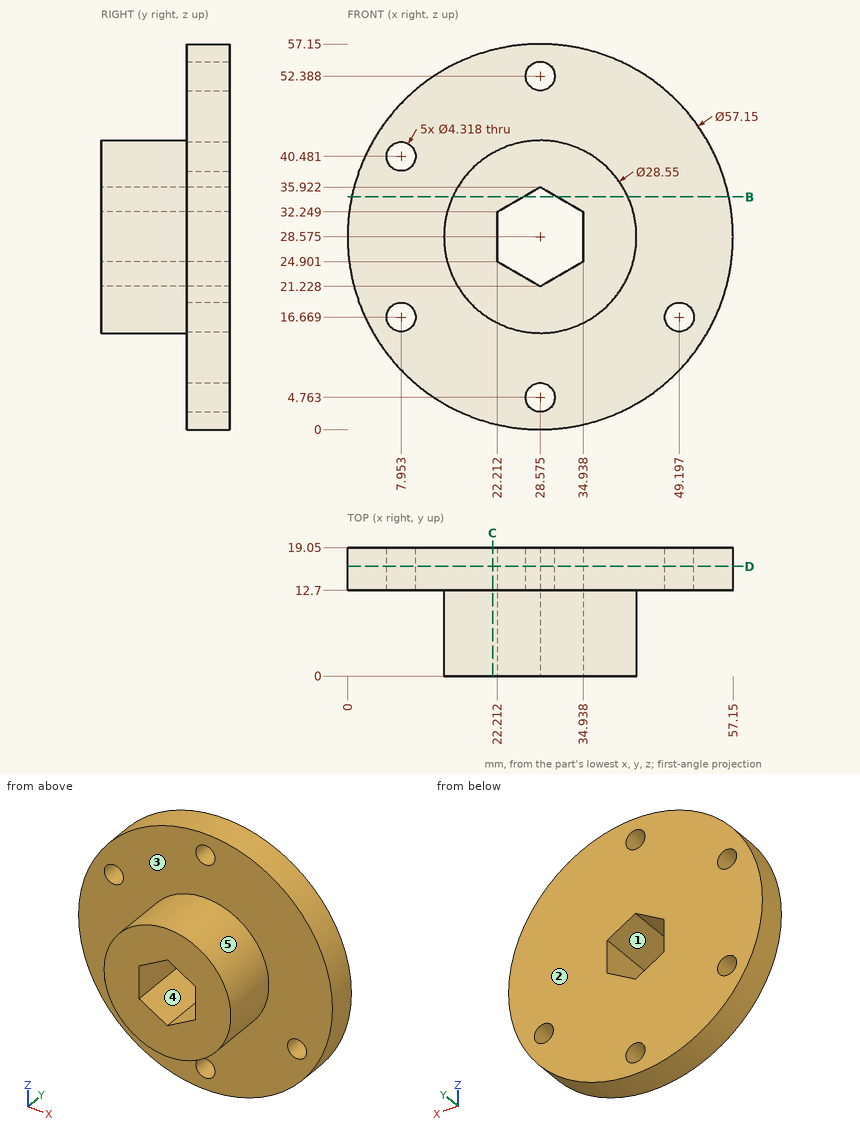
For this review, use the dimensioned drawing (mm, ordinates from the lowest corner) and the shaded views. A direction names the side the tool comes from. Coordinates: 2 decimals unless noted, no trailing zeros. Loops run counter-clockwise (first coordinate to the right, second up) from the corner with the lowest first, then second, coordinate; pieces in that order, holes last. Notation, with made-up numbers: (45, 34) - (53, 34) arc R29 cw to (53, 63) - close; hole circle Ø9 at (-35, -21.75). An arc over 180 degrees is marked (long way). Use one line per item in the form item = value. Start each with the question number.
1) Take a section at B-B (z = 34.5). State the section outline as (x, y) points.
2) Take a section at C-C (x = 21.5). State the section outline as (y, z) points.
3) To check wall thickness, follow probe 1 along X at (y, z) = (1.25, 30); probe 2 along X at (y, z) = (17.5, 29); probe 3 along Y at (x, z) = (30, 44). State the ranges of each line that lie inside material, in increasing order. Write a range as from..to.
4) Take a section at D-D (y = 16.25). State how many separate pieces and enclosed holes the cut face has, plus the area to 3 significant figures.
5) For the marked faces 1 and 2, list the 3-axis set-ups (+Z, -Z, +X, -X, +Y, -Y) from which the entire face can be reached by the end or side of a thin tool; tool diameter is ignored.
6) For pin 1 (1 mm diameter, centred on x = 24, y = 8, fed in from +Z) (1 decimal); pin 2 (1 mm diameter, centred on y = 8, z = 42, fed in from +X) (1 decimal); pin 3 (3 mm diameter, centred on x = 34.5, y = 6.5, fed in from -Z), all flat-tipped, find the tip position at first contact; note any pin that passes through.
7) Draft analysis for pull direction Z (two halves, no side actions). For the marked faces 3, 4 and 5, state which applies: released by +Z, released by -Z, zero draft, split by the parting line, or undercut.
From the geometry:
q1.outline = (0.62, 12.7) - (15.59, 12.7) - (15.59, 0) - (26.11, 0) - (26.11, 19.05) - (0.62, 19.05) - close; (31.04, 0) - (41.56, 0) - (41.56, 12.7) - (56.53, 12.7) - (56.53, 19.05) - (31.04, 19.05) - close
q2.outline = (0, 16.18) - (12.7, 16.18) - (12.7, 0.89) - (19.05, 0.89) - (19.05, 56.26) - (12.7, 56.26) - (12.7, 40.97) - (0, 40.97) - close
q3.probe_1 = 14.37..22.21, 34.94..42.78
q3.probe_2 = 0..22.21, 34.94..57.15
q3.probe_3 = 12.7..19.05
q4.separate_pieces = 1
q4.enclosed_holes = 6
q4.area = 2,350 mm2
q5.face_1 = +Y, -Y
q5.face_2 = +Z, -Z, +X, -X, +Y
q6.pin_1 = 42.3
q6.pin_2 = 34.6
q6.pin_3 = 15
q7.face_3 = zero draft
q7.face_4 = undercut
q7.face_5 = split by the parting line
